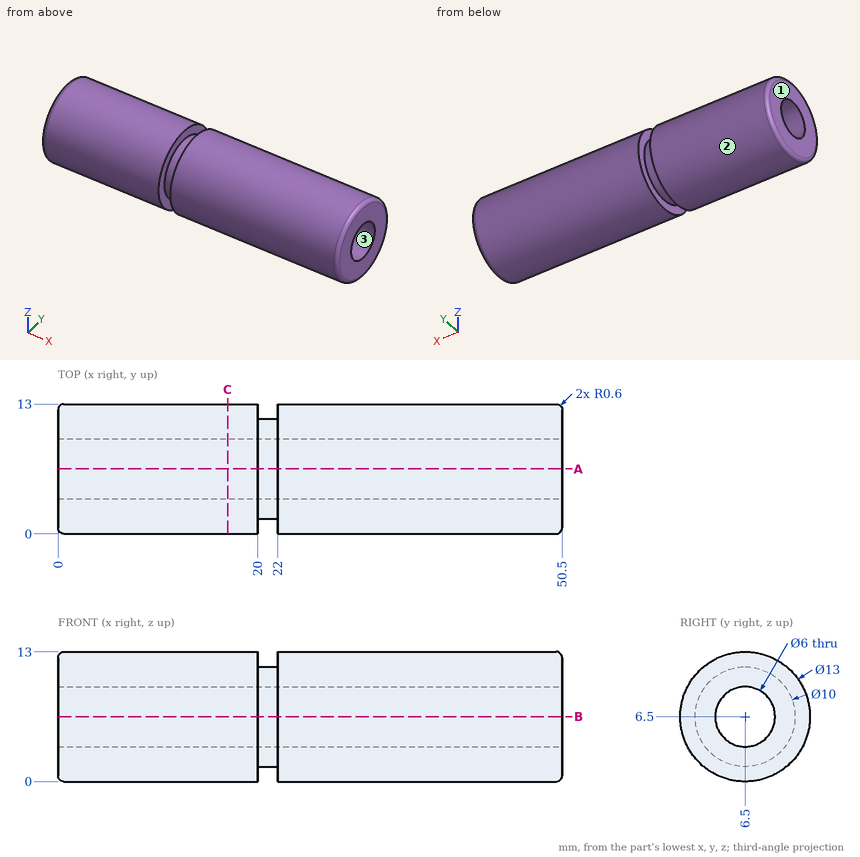
Part print with two shaded views. Sizes in mm from the minimum x, y, z corner. Round coordinates to 2 decimals unless told otherwise and drop trailing zeros. Loops run counter-clockwise (first coordinate to the right, second up) from the corner with the lowest first, then second, coordinate; pieces in that order, holes last. Notation, with made-up numbers: M 40,89.25 L 51,89.25 A13 ccw 51,108.25 Z; hole C 65.25,65 d10. An arc over 180 degrees is marked long. Put each result on its own line as item: value. Start each with the question number.
Item 1: Drill centre lines: line 1 along Y through (x, z) = (13, 6.5); line 2 along X through (y, z) = (10.75, 9.5); line 3 along Z through (x, y) = (23, 6.25). Where is each one in solid material? Low to high.
Item 2: Mould opens along Z. For the marked faces 1, 2 and 3 say: released by +Z, released by -Z, zero draft, split by the parting line, or undercut.
Item 3: Cut at A-A (y = 6.5). List the corners of the cut face in (x, z), then the cut area to 3 significant figures.
Item 4: Drop flat-ended pins along their axis: P1, Ø2, axis at x = 20.5, y = 3.5, coming from the +Z side; P2, Ø3, axis at x = 13, z = 8.5, coming from the -Y side; P3, Ø1.5, axis at x = 34.5, z = 1.5, coming from the -Y side. Give the stop position or say it passes through.
Item 5: Cut at C-C (x = 17). List the corners of the cut face in (y, z).
Answer block:
1. line 1: 0 to 3.5, 9.5 to 13
1. line 2: 0 to 20, 22 to 50.5
1. line 3: 0 to 3.51, 9.49 to 13
2. face 1: zero draft
2. face 2: split by the parting line
2. face 3: undercut
3. outline: M 0,0.6 A0.6 ccw 0.6,0 L 20,0 L 20,1.5 L 22,1.5 L 22,0 L 49.9,0 A0.6 ccw 50.5,0.6 L 50.5,3.5 L 0,3.5 Z; M 0,9.5 L 50.5,9.5 L 50.5,12.4 A0.6 ccw 49.9,13 L 22,13 L 22,11.5 L 20,11.5 L 20,13 L 0.6,13 A0.6 ccw 0,12.4 Z
3. area: 347 mm2
4. P1: z = 12.64
4. P2: y = 0.02
4. P3: y = 1.58
5. outline: C 6.5,6.5 d13; hole C 6.5,6.5 d6
